Design review of the part shown in the three views and the two pictorial views. Dimensions are in mm from the part's minimum x, y and z. Round coordinates to 2 decimals unless told otherwise and drop trailing zeros. Loops run counter-clockwise (first coordinate to the right, second up) from the corner with the lowest first, then second, coordinate; pieces in that order, holes last. Notation, with made-up numbers: M 25.5,47.5 L 55.5,47.5 A9 ccw 55.5,63.5 Z; hole C -39.5,43 d8. An arc over 180 degrees is marked long. Answer as CSV lines item,"result". Start each with the question number.
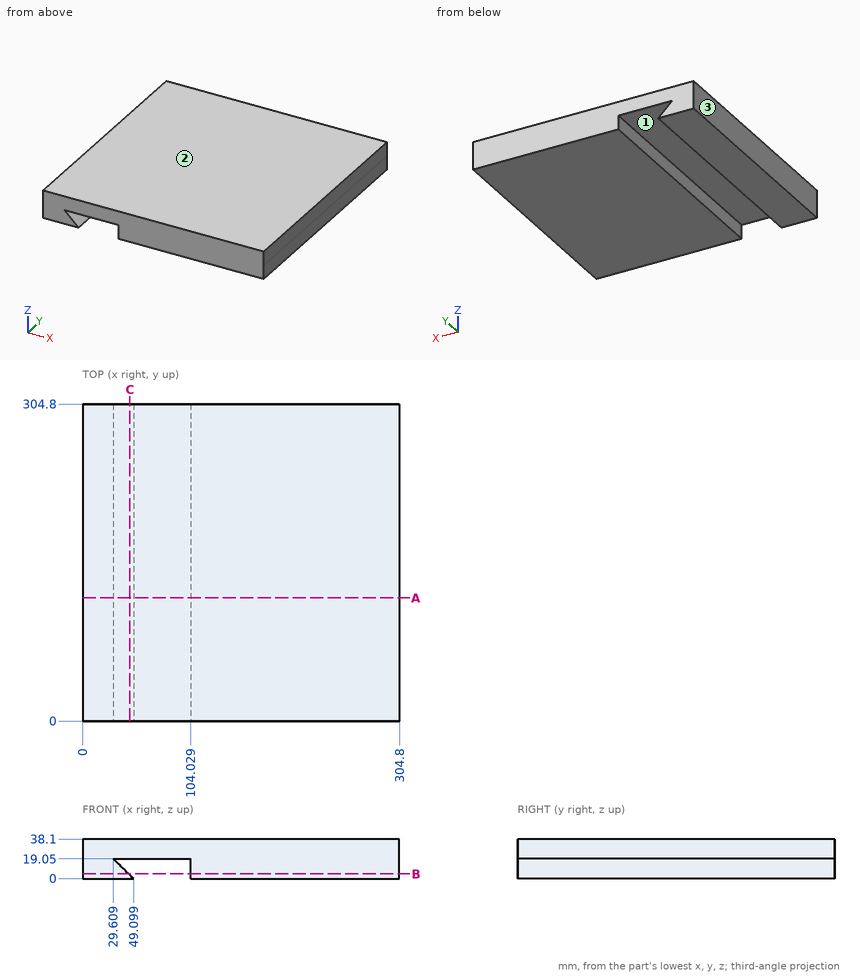
Item 1: Insertion check: pin 1 Ø3 at (x, z) = (48.5, 18) entering from +Y; pin 2 Ø22.5 at (x, y) = (78, 206.5) entering from -Z. Each pin has a flat end and moves straight along its axis. Give the tip position at first contact, or say it passes through.
Item 2: Consider section B-B, the plane z = 4.5. Write out the cut boundary in (x, y) (1 decimal), then the cut area to 3 significant figures.
Item 3: The part is to be moulded in two halves that separate along X. For the marked faces 1, 2 and 3, say which applies: +X half, -X half, draft (parallel to the pull), parting line (faces both ways), or undercut.
Item 4: To check wall thickness, follow line 1 (X direction, y = 280, z = 19); line 2 (Z direction, x = 89.5, y = 25); line 3 (X direction, y = 151.5, z = 6). State the ranges of each line that lie inside material, in increasing order.
Item 5: Consider section C-C, the plane x = 45.5. Write out the cut boundary in (y, z), then the cut area to 3 significant figures.
Item 6: Consider section A-A, the plane y = 118.5. Write out the cut boundary in (x, z), then the cut area to 3 significant figures.
Found:
1,pin 1,"stops at y = 304.8"
1,pin 2,"stops at z = 19.05"
2,outline,"M 0,0 L 44.5,0 L 44.5,304.8 L 0,304.8 Z; M 104,0 L 304.8,0 L 304.8,304.8 L 104,304.8 Z"
2,area,"74,800 mm^2"
3,face 1,"undercut"
3,face 2,"draft"
3,face 3,"-X half"
4,line 1,"x = 0 to 29.66, 104.03 to 304.8"
4,line 2,"z = 19.05 to 38.1"
4,line 3,"x = 0 to 42.96, 104.03 to 304.8"
5,outline,"M 0,0 L 304.8,0 L 304.8,3.52 L 0,3.52 Z; M 0,19.05 L 304.8,19.05 L 304.8,38.1 L 0,38.1 Z"
5,area,"6,880 mm^2"
6,outline,"M 0,0 L 49.1,0 L 29.61,19.05 L 104.03,19.05 L 104.03,0 L 304.8,0 L 304.8,38.1 L 0,38.1 Z"
6,area,"10,400 mm^2"
